Verification items for the finished model (mm, model axes). Round coordinates to 2 decimals unless told otherwise and drop trailing zeros. Write each loop counter-clockwise with the first axis right and the second up, starting at its lowest first coordinate (ties: lowest second). Pieces come first, ordered by that corner, then holes. Notation, with made-up numbers: (75.25, -18.5) -> (79.25, -18.5) arc R10 ccw to (79.25, -3.5) -> close; hole circle Ø9 at (12.25, 13.5). An arc over 180 degrees is marked (long way). Answer as a JSON object with one key per item and string values. Group by question number.
(1) Sectioned sample at B-B on y = 3.75. Record the cut outline in (x, z).
(2) Sectioned sample at A-A on x = 3. Record the cut outline in (y, z).
(3) Scan lines: L1, parallel to Y at x = 64, z = 24.5; L2, parallel to X at y = 3, z = 24; L3, parallel to Y at x = 65, z = 17. Record each from-to range of solid material in increasing order. Write a range as from..to.
(4) Gauge pin test, flat end, axial feed: pin 1 Ø1.8 at (x, y) = (3, 37.25) entering from +Z. Record the tip position at first contact, or that the pin passes through.
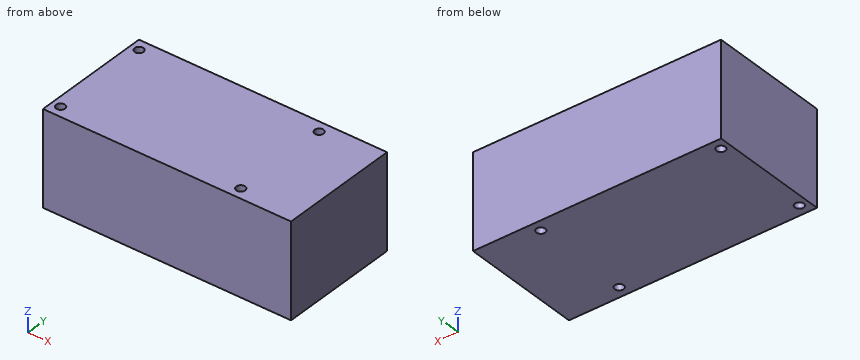
```python
from build123d import *

# Parameters (mm, degrees)
SKETCH_1_W          = 84
SKETCH_1_H          = 41
EXTRUDE_1_DEPTH     = 32
SKETCH_2_R          = 1.5
CUT_EXTRUDE_1_DEPTH = 32


with BuildPart() as part:
    # 草图1 → 凸台-拉伸1 (new body)
    with BuildSketch(Plane.XY):
        with Locations((42, 20.5)):
            Rectangle(SKETCH_1_W, SKETCH_1_H)
    extrude(amount=EXTRUDE_1_DEPTH)

    # 草图2 → 切除-拉伸1 (cut)
    with BuildSketch(Plane.XY.offset(32)):
        with Locations((3, 3.75)):
            Circle(SKETCH_2_R)
        with Locations((64, 3.75)):
            Circle(SKETCH_2_R)
        with Locations(Location((64, 37.25, 0), (0, 0, 180))):
            Circle(SKETCH_2_R)
        with Locations(Location((3, 37.25, 0), (0, 0, 180))):
            Circle(SKETCH_2_R)
    extrude(amount=-CUT_EXTRUDE_1_DEPTH, mode=Mode.SUBTRACT)


solid = part.part
```
Computed values:
{
 "1": {"outline": "(0, 0) -> (1.5, 0) -> (1.5, 32) -> (0, 32) -> close; (4.5, 0) -> (62.5, 0) -> (62.5, 32) -> (4.5, 32) -> close; (65.5, 0) -> (84, 0) -> (84, 32) -> (65.5, 32) -> close"},
 "2": {"outline": "(0, 0) -> (2.25, 0) -> (2.25, 32) -> (0, 32) -> close; (5.25, 0) -> (35.75, 0) -> (35.75, 32) -> (5.25, 32) -> close; (38.75, 0) -> (41, 0) -> (41, 32) -> (38.75, 32) -> close"},
 "3": {"L1": "0..2.25, 5.25..35.75, 38.75..41", "L2": "0..1.7, 4.3..62.7, 65.3..84", "L3": "0..2.63, 4.87..36.13, 38.37..41"},
 "4": {"pin 1": "through"}
}
